```python
from build123d import *

# Parameters (mm, degrees)
F0_W      = 44.45
F0_H      = 25.4
F1_DEPTH  = 12.7
F2_R      = 12.7
F3_DEPTH  = 12.7
F4_W      = 12.7
F4_H      = 25.4
F5_DEPTH  = 25.4
F6_R      = 12.7
F7_DEPTH  = 12.7
F8_R      = 6.35
F9_DEPTH  = 12.7
F10_W     = 12.7
F10_H     = 21.287267
F11_DEPTH = 25.4
F12_R     = 6.35
F13_DEPTH = 25.4


with BuildPart() as f1:
    # F0 (on Top) → F1 (new body)
    with BuildSketch(Plane.XY):
        with Locations((22.225, 12.7)):
            Rectangle(F0_W, F0_H)
    extrude(amount=F1_DEPTH)

    # F2 (on face) → F3 (join)
    with BuildSketch(Plane.XY.offset(12.7)):
        with Locations((44.45, 12.7)):
            Circle(F2_R)
    extrude(amount=-F3_DEPTH)

    # F4 (on face) → F5 (join)
    with BuildSketch(Plane.XY.offset(12.7)):
        with Locations((6.35, 12.7)):
            Rectangle(F4_W, F4_H)
    extrude(amount=F5_DEPTH)

    # F6 (on face) → F7 (join)
    with BuildSketch(Plane(origin=(0, 0, 0), x_dir=(0, -1, 0), z_dir=(-1, 0, 0))):
        with Locations((-12.7, 38.1)):
            Circle(F6_R)
    extrude(amount=-F7_DEPTH)

    # F8 (on face) → F9 (cut)
    with BuildSketch(Plane(origin=(0, 0, 0), x_dir=(0, -1, 0), z_dir=(-1, 0, 0))):
        with Locations((-12.7, 38.1)):
            Circle(F8_R)
    extrude(amount=-F9_DEPTH, mode=Mode.SUBTRACT)

    # F10 (on face) → F11 (cut)
    with BuildSketch(Plane.YZ.offset(12.7)):
        with Locations((12.7, 48.743634)):
            Rectangle(F10_W, F10_H)
    extrude(amount=-F11_DEPTH, mode=Mode.SUBTRACT)

    # F12 (on face) → F13 (cut)
    with BuildSketch(Plane.XY.offset(12.7)):
        with Locations((44.45, 12.7)):
            Circle(F12_R)
        with Locations((25.4, 12.7)):
            Circle(F12_R)
    extrude(amount=-F13_DEPTH, mode=Mode.SUBTRACT)


solid = f1.part
```
Geometry check sheet. Reference: the model listing, model coordinates, mm. A direction names the side the tool comes from. Coordinates: 2 decimals unless noted, no trailing zeros. Order: outer loops, then holes, each group sorted by start corner. A loop starts at its lowest first (then second) coordinate and runs counter-clockwise, first axis right, second up. Notation, with made-up numbers: M 17,73 L 37,73 A33 ccw 37,102 Z; hole C 62,61.5 d8. An arc over 180 degrees is marked long. Answer as a JSON object with one key per item and string values.
Q1. Cross-section at A-A on y = 12.7. Record the cut outline in (x, z).
Results are:
{"outline": "M 0,0 L 19.05,0 L 19.05,12.7 L 12.7,12.7 L 12.7,31.75 L 0,31.75 Z; M 31.75,0 L 38.1,0 L 38.1,12.7 L 31.75,12.7 Z; M 50.8,0 L 57.15,0 L 57.15,12.7 L 50.8,12.7 Z"}
Q2. Tool access check on faces 1 (the flat face through (12.7, 13, 27)), 2 (the cylindrical face through (6.26, 23.65, 44.53)), 3 (the flat face through (6, 19.05, 44)). Record the directions out of +Z, -Z, +X, -X, +Y, -Y that give a thin tool (end or side, any length) a straight path to the whole face; none if there is none.
Results are:
{"face 1": "+Z, +X, +Y, -Y", "face 2": "+Z, +X, -X, +Y", "face 3": "+Z, +X, -X"}
Q3. Cross-section at D-D on z = 11. Record the cut outline in (x, y).
Results are:
{"outline": "M 0,0 L 44.45,0 A12.7 ccw 44.45,25.4 L 0,25.4 Z; hole C 25.4,12.7 d12.7; hole C 44.45,12.7 d12.7"}
Q4. Cross-section at B-B on x = 25.4. Record the cut outline in (y, z), and give its area (3 significant figures).
Results are:
{"outline": "M 0,0 L 6.35,0 L 6.35,12.7 L 0,12.7 Z; M 19.05,0 L 25.4,0 L 25.4,12.7 L 19.05,12.7 Z", "area": "161 mm²"}
Q5. Cross-section at C-C on z = 37. Record the cut outline in (x, y), and give its area (3 significant figures).
Results are:
{"outline": "M 0,0 L 12.7,0 L 12.7,6.45 L 0,6.45 Z; M 0,18.95 L 12.7,18.95 L 12.7,25.4 L 0,25.4 Z", "area": "164 mm²"}
Q6. Release check for a two-part mould opening along X. For faces 4 (the cylindrical face through (57.147, 12.421, 6.439)), 5 (the cylindrical face through (20.72, 16.99, 6.44)), 6 (the flat face through (6, 6.35, 44)), 7 (the cylindrical face through (50.507, 14.607, 6.439)) record: released by +X, released by -X, zero draft, split by the parting line, or undercut.
Results are:
{"face 4": "released by +X", "face 5": "undercut", "face 6": "zero draft", "face 7": "undercut"}
Q7. Depth check by flat-ended pin: pin 1 Ø3 at (y, z) = (13, 26.5) entering from -X; pin 2 Ø3.5 at (x, z) = (8.5, 42.5) entering from +Y; pin 3 Ø10 at (y, z) = (16.5, 16.5) entering from +X. Enter the tip coordinate at first touch or a pass-through.
Results are:
{"pin 1": "stops at x = 0", "pin 2": "stops at y = 25.12", "pin 3": "stops at x = 57.14"}
Q8. Scan lines: line 1 (Y direction, x = 25.4, z = 7.5); line 2 (Z direction, x = 46.5, y = 20). Record each from-to range of solid material in increasing order.
Results are:
{"line 1": "y = 0 to 6.35, 19.05 to 25.4", "line 2": "z = 0 to 12.7"}
